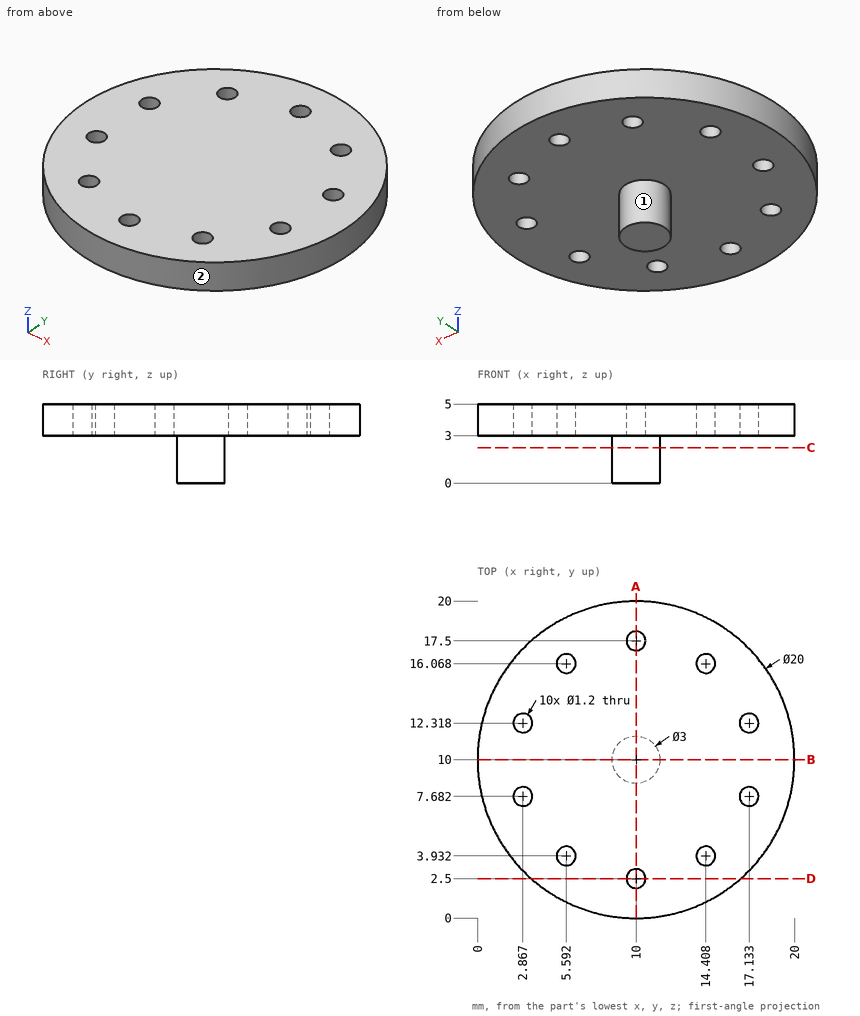
Verification items for this drawing (mm, ordinates from the low corner). A direction names the side the tool comes from. Coordinates: 2 decimals unless noted, no trailing zeros. Order: outer loops, then holes, each group sorted by start corner. A loop starts at its lowest first (then second) coordinate and runs counter-clockwise, first axis right, second up.
Q1. Sectioned sample at A-A on x = 10. Record the cut outline in (y, z).
Reply:
outline: (0, 3) - (1.9, 3) - (1.9, 5) - (0, 5) - close; (3.1, 3) - (8.5, 3) - (8.5, 0) - (11.5, 0) - (11.5, 3) - (16.9, 3) - (16.9, 5) - (3.1, 5) - close; (18.1, 3) - (20, 3) - (20, 5) - (18.1, 5) - close
Q2. Sectioned sample at D-D on y = 2.5. Record the cut outline in (x, z) (1 decimal).
Reply:
outline: (3.4, 3) - (9.4, 3) - (9.4, 5) - (3.4, 5) - close; (10.6, 3) - (16.6, 3) - (16.6, 5) - (10.6, 5) - close
Q3. Sectioned sample at C-C on z = 2.25. Record the cut outline in (x, y).
Reply:
outline: circle Ø3 at (10, 10)
Q4. Sectioned sample at B-B on y = 10. Record the cut outline in (x, z).
Reply:
outline: (0, 3) - (8.5, 3) - (8.5, 0) - (11.5, 0) - (11.5, 3) - (20, 3) - (20, 5) - (0, 5) - close
Q5. Thickness scan on probe 1 along Y at (x, z) = (10, 3.85); probe 2 along Y at (x, z) = (14.25, 4.6) (1 decimal); probe 3 along Z at (x, y) = (13.25, 15.25). Record the ranges inside material, lowest first.
Reply:
probe 1: y = 0 to 1.9, 3.1 to 16.9, 18.1 to 20
probe 2: y = 0.9 to 3.4, 4.5 to 15.5, 16.6 to 19.1
probe 3: z = 3 to 5
Q6. Tool access check on the marked faces 1 and 2. Record the directions out of +Z, -Z, +X, -X, +Y, -Y that give a thin tool (end or side, any length) a straight path to the whole face; none if there is none.
Reply:
face 1: -Z
face 2: +Z, -Z
Q7. Depth check by flat-ended pin: pin 1 Ø1.1 at (x, y) = (2.87, 7.68) entering from +Z; pin 2 Ø3 at (y, z) = (12, 3) entering from -X; pin 3 Ø3 at (x, z) = (10.5, 2) entering from +Y; pin 4 Ø1.6 at (x, y) = (14.41, 3.93) entering from -Z. Enter the tip coordinate at first touch or a pass-through.
Reply:
pin 1: passes through
pin 2: stops at x = 0.01
pin 3: stops at y = 20
pin 4: stops at z = 3
